Solid Edge part; units mm, degrees
sketch "Sketch1" plane through (0, 0, 0) normal (0, 0, 1) x (1, 0, 0)
  line L0 (-3.574, 68.8217) -> (-3.574, 66.1655)
  line L1 (-3.574, 66.1655) -> (-1.1455, 66.1655)
  line L2 (-1.1455, 66.1655) -> (-1.1455, 68.594)
  line L3 (-1.1455, 68.594) -> (1.283, 68.594)
  line L4 (1.283, 68.594) -> (0.7116, 70.8796)
  line L5 (0.7116, 70.8796) -> (-2.6169, 70.0475)
  line L6 (-2.6169, 70.0475) -> (-3.574, 68.8217)
revolve "RevolvedProtrusion1" add sketch "Sketch1" angle 360 about axis through (50, 0, 0) along (-1, 0, 0)
The listing builds one solid part. Answer for the finished solid, in the listing's coordinates (mm). A direction names the side the tool comes from. Give positions to 0.01 mm unless a question says otherwise; leave off trailing zeros. Order: outer loops, then holes, each group sorted by start corner. A loop starts at its lowest first (then second) coordinate and runs counter-clockwise, first axis right, second up. Notation, with made-up numbers: (-12.75, 25.5) -> (6.25, 25.5) arc R15 ccw to (6.25, 42.5) -> close; hole circle Ø3 at (51, -11.5). An arc over 180 degrees is marked (long way). Write each question's results on one line, items separated by ' | '.
Q1. Straight lines are drawn through the part: probe 1 along Y at (x, z) = (0.55, 0); probe 2 along Y at (x, z) = (0.1, 7.5); probe 3 along Z at (x, y) = (0.65, 0). For each, find the intervals that lie inside material, in ascending order. Write a range as from..to.
Checked values:
probe 1: y = -70.84..-68.59, 68.59..70.84 | probe 2: y = -70.33..-68.18, 68.18..70.33 | probe 3: z = -70.86..-68.59, 68.59..70.86
Q2. Which of the six approach directions +Z, -Z, +X, -X, +Y, -Y give full straight-line access (tool end or side, diameter ignored) to faces 1 (the face through (0.086, -14.87, -66.963)), 2 (the face through (-2.3, -14.3, -64.6))?
Checked values:
face 1: +X | face 2: +X, -X
Q3. Determine the mould class of faces 3 (the face through (-1.146, -36, -56)), 4 (the face through (-2.409, -9.126, 69.503)), 5 (the face through (-3.574, -36, -56)) for opening direction Y: pulls with the +Y half, pulls with the -Y half, needs draft (parallel to the pull), parting line crosses it, or undercut.
Checked values:
face 3: undercut | face 4: parting line crosses it | face 5: needs draft
Q4. The part is cut by section A-A, the plane y = 0. Give the vertices of the cut face in (x, z), and give its area (3 significant figures).
Checked values:
outline: (-3.57, -68.82) -> (-2.62, -70.05) -> (0.71, -70.88) -> (1.28, -68.59) -> (-1.15, -68.59) -> (-1.15, -66.17) -> (-3.57, -66.17) -> close; (-3.57, 66.17) -> (-1.15, 66.17) -> (-1.15, 68.59) -> (1.28, 68.59) -> (0.71, 70.88) -> (-2.62, 70.05) -> (-3.57, 68.82) -> close | area: 27.2 mm^2
